Part model, mm, in its own coordinate system. Face numbers are marked on the shaded views. A direction names the side the tool comes from. Give positions to 0.01 mm unless a question says otherwise; leave off trailing zeros. Loops run counter-clockwise (first coordinate to the right, second up) from the corner with the lowest first, then second, coordinate; pieces in that order, holes last. Notation, with made-up numbers: M 49,10.5 L 105,10.5 A23 ccw 105,29.5 Z; hole C 68,35 d9. An arc over 180 degrees is marked long. Put each result on its own line as item: value. Start each with the question number.
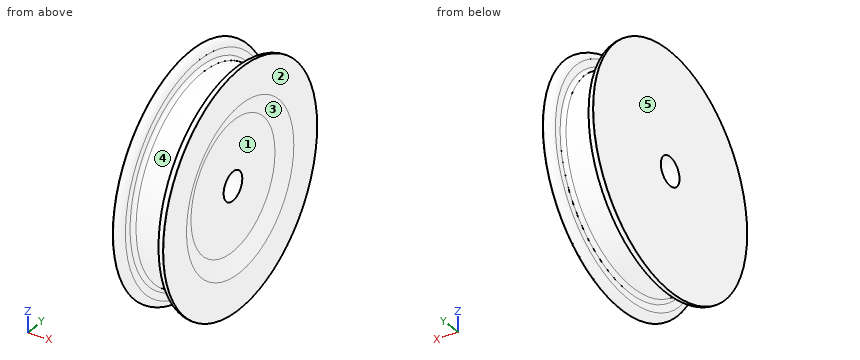
```python
from build123d import *

# Parameters (mm, degrees)
FILLET1_R = 0.5


with BuildPart() as part:
    # Sketch1 → Revolve1 (revolve)
    with BuildSketch(Plane.XY):
        with BuildLine():
            Line((1.75, 8.25), (1.2, 8.25))
            Line((1.2, 8.25), (1.2, 7.25))
            ThreePointArc((1.2, 7.25), (1.126776695, 7.073223305), (0.95, 7))
            Line((0.95, 7), (-0.95, 7))
            ThreePointArc((-0.95, 7), (-1.126776695, 7.073223305), (-1.2, 7.25))
            Line((-1.2, 7.25), (-1.2, 8.25))
            Line((-1.2, 8.25), (-1.75, 8.25))
            Line((-1.75, 8.25), (-1.75, 1))
            Line((-1.75, 1), (1.25, 1))
            Line((1.25, 1), (1.25, 4.5))
            Line((1.25, 4.5), (1.75, 5.75))
            Line((1.75, 5.75), (1.75, 8.25))
        make_face()
    revolve(axis=Axis((0, 0, 0), (1, 0, 0)))

    # Fillet1
    fillet1_edges = [part.edges().sort_by_distance(p)[0] for p in [
        (1.2, -8.25, 0),
        (-1.2, -8.25, 0),
    ]]
    fillet(fillet1_edges, radius=FILLET1_R)


solid = part.part
```
1) Mould opens along Z. For the marked faces 3, 4 and 5 say: +Z half, -Z half, draft (parallel to the pull), parting line (faces both ways), or undercut.
2) Band-saw the part on A-A on y = 0. Give the cut face in (x, z).
3) Pin check, flat tips, straight feed: pin 1 Ø2 at (x, y) = (1, -5.5) entering from -Z; pin 2 Ø7 at (y, z) = (1, -1.5) entering from +X; pin 3 Ø4.5 at (y, z) = (0.5, -2) entering from +X. Stop position of each tip, or through.
4) Wall check: L1, parallel to Z at x = -0.2, y = 0; L2, parallel to X at y = -3.25, z = -6.5; L3, parallel to X at y = 4.75, z = -6.5. Give the ranges that are in metal, low to high.
5) Band-saw the part on C-C on x = -0.6. Give the cut face in (y, z), then the cut area to 3 significant figures.
6) Which spindle directions (+Z, -Z, +X, -X, +Y, -Y) get a long thin tool onto all of the face, cutting with end or side? Do the marked faces 1 and 2. Say none if no direction does.
Evaluation:
1. face 3: undercut
1. face 4: parting line
1. face 5: draft
2. outline: M -1.75,-8.25 L -1.7,-8.25 A0.5 ccw -1.2,-7.75 L -1.2,-7.25 A0.25 cw -0.95,-7 L 0.95,-7 A0.25 cw 1.2,-7.25 L 1.2,-7.75 A0.5 ccw 1.7,-8.25 L 1.75,-8.25 L 1.75,-5.75 L 1.25,-4.5 L 1.25,-1 L -1.75,-1 Z; M -1.75,1 L 1.25,1 L 1.25,4.5 L 1.75,5.75 L 1.75,8.25 L 1.7,8.25 A0.5 ccw 1.2,7.75 L 1.2,7.25 A0.25 cw 0.95,7 L -0.95,7 A0.25 cw -1.2,7.25 L -1.2,7.75 A0.5 ccw -1.7,8.25 L -1.75,8.25 Z
3. pin 1: z = -6.78
3. pin 2: x = 1.57
3. pin 3: x = 1.25
4. L1: -7 to -1, 1 to 7
4. L2: -1.75 to -1.2, 1.2 to 1.75
4. L3: -1.75 to -1.3, 1.3 to 1.75
5. outline: C 0,0 d14; hole C 0,0 d2
5. area: 151 mm2
6. face 1: +X
6. face 2: +Z, -Z, +X, +Y, -Y
